Geometry check sheet. Reference: the model listing, model coordinates, mm. A direction names the side the tool comes from. Round coordinates to 2 decimals unless told otherwise and drop trailing zeros. Loops run counter-clockwise (first coordinate to the right, second up) from the corner with the lowest first, then second, coordinate; pieces in that order, holes last. Notation, with made-up numbers: (39.25, 84.25) -> (58.25, 84.25) arc R27 ccw to (58.25, 121.25) -> close; hole circle Ø4 at (72, 26). An arc over 180 degrees is marked (long way). Use a Markdown table: item, result. Add a question column.
Q1. Gauge pin test, flat ends, axial feed: P1, Ø3, axis at x = 16.5, y = -2, coming from the -Z side; P2, Ø1.9, axis at y = -2, z = -54, coming from the -X side; P3, Ø2, axis at y = -2.5, z = 5.5, coming from the +X side. Record the tip position at first contact, or that the pin passes through.
Q2. Set-up check for faces 5 (the face through (-25, -3, 0)), 6 (the face through (-9.75, -3, -53)), 7 (the face through (25, -3, 0)): record each of +Z, -Z, +X, -X, +Y, -Y from which the full face is reachable in a straight line by a thin tool's end or side.
Q3. Release check for a two-part mould opening along Z. For faces 1 (the face through (9.75, -3, -53)), 2 (the face through (-28, -3, 10)), 3 (the face through (-28, -3, -10)), 4 (the face through (-21, -3, -50)) record: released by +Z, released by -Z, zero draft, split by the parting line, or undercut.
Q4. Material ranges on L1, parallel to Z at x = -28, y = -3; L2, parallel to Z at x = 22.5, y = -1.5; L3, parallel to X at y = -3.75, z = 3, recorded low to high.
Q5. Sectioned sample at D-D, the plane x = -17. Enter the section's corners in (y, z), then the cut area to 3 significant figures.
Q6. Sectioned sample at C-C, the plane z = -5. Enter the section's corners in (x, y), then the cut area to 4 significant figures.
Q7. Sectioned sample at B-B, the plane y = -4.75. Enter the section's corners in (x, z), then the cut area to 3 significant figures.
Q8. Sectioned sample at A-A, the plane x = -27. Enter the section's corners in (y, z).
```python
from build123d import *

# Parameters (mm, degrees)
F0_W     = 6.35
F0_H     = 40
F0_W_2   = 19.5
F0_H_2   = 6.35
F1_DEPTH = 6.35


with BuildPart() as f1:
    # F0 (on Front) → F1 (new body)
    with BuildSketch(Plane.XZ):
        Polygon((25, 10), (25, 50), (-25, 50), (-25, 10), (-25, -10), (-25, -50), (-9.75, -50), (9.75, -50), (25, -50), (25, -10), align=None)
        with Locations((28.175, 30)):
            Rectangle(F0_W, F0_H)
        with Locations((-28.175, 30)):
            Rectangle(F0_W, F0_H)
        with Locations((28.175, -30)):
            Rectangle(F0_W, F0_H)
        with Locations((-28.175, -30)):
            Rectangle(F0_W, F0_H)
        with Locations((0, -53.175)):
            Rectangle(F0_W_2, F0_H_2)
    extrude(amount=F1_DEPTH)


solid = f1.part
```
Values:
| question | item | result |
|---|---|---|
| 1 | P1 | z = -50 |
| 1 | P2 | x = -9.75 |
| 1 | P3 | x = 25 |
| 2 | face 5 | -X, +Y, -Y |
| 2 | face 6 | -Z, -X, +Y, -Y |
| 2 | face 7 | +X, +Y, -Y |
| 3 | face 1 | zero draft |
| 3 | face 2 | undercut |
| 3 | face 3 | undercut |
| 3 | face 4 | released by -Z |
| 4 | L1 | -50 to -10, 10 to 50 |
| 4 | L2 | -50 to 50 |
| 4 | L3 | -25 to 25 |
| 5 | outline | (-6.35, -50) -> (0, -50) -> (0, 50) -> (-6.35, 50) -> close |
| 5 | area | 635 mm^2 |
| 6 | outline | (-25, -6.35) -> (25, -6.35) -> (25, 0) -> (-25, 0) -> close |
| 6 | area | 317.5 mm^2 |
| 7 | outline | (-31.35, -50) -> (-9.75, -50) -> (-9.75, -56.35) -> (9.75, -56.35) -> (9.75, -50) -> (31.35, -50) -> (31.35, -10) -> (25, -10) -> (25, 10) -> (31.35, 10) -> (31.35, 50) -> (-31.35, 50) -> (-31.35, 10) -> (-25, 10) -> (-25, -10) -> (-31.35, -10) -> close |
| 7 | area | 6,140 mm^2 |
| 8 | outline | (-6.35, -50) -> (0, -50) -> (0, -10) -> (-6.35, -10) -> close; (-6.35, 10) -> (0, 10) -> (0, 50) -> (-6.35, 50) -> close |
